Read the model definition and answer for the solid it produces. Units are mm, in the model's axes. A direction names the side the tool comes from. Coordinates: 2 decimals unless noted, no trailing zeros. Loops run counter-clockwise (first coordinate to the right, second up) from the corner with the lowest first, then second, coordinate; pieces in that order, holes last. Notation, with made-up numbers: M 13,27 L 45,27 A21 ccw 45,32 Z; hole C 34,39 d3. An arc over 180 degrees is marked long. Put each result on its own line as item: value.
from build123d import *

# Parameters (mm, degrees)
CROQUIS1_R              = 11
CROQUIS1_R_2            = 6
SALIENTE_EXTRUIR1_DEPTH = 25
CROQUIS2_W              = 6
CROQUIS2_H              = 22
CORTAR_EXTRUIR1_DEPTH   = 25
CROQUIS3_R              = 11
CROQUIS3_R_2            = 8.5
SALIENTE_EXTRUIR2_DEPTH = 25
SALIENTE_EXTRUIR3_DEPTH = 10
SALIENTE_EXTRUIR4_DEPTH = 10
CROQUIS9_R              = 11
CROQUIS9_R_2            = 8.5
SALIENTE_EXTRUIR5_DEPTH = 10
CROQUIS13_R             = 11
CROQUIS13_R_2           = 6
SALIENTE_EXTRUIR6_DEPTH = 5
CROQUIS14_W             = 6
CROQUIS14_H             = 22
CORTAR_EXTRUIR2_DEPTH   = 5
CROQUIS15_R             = 11
CROQUIS15_R_2           = 8.5
SALIENTE_EXTRUIR7_DEPTH = 5


with BuildPart() as part:
    # Croquis1 → Saliente-Extruir1 (new body)
    with BuildSketch(Plane.XY):
        Circle(CROQUIS1_R)
        Circle(CROQUIS1_R_2, mode=Mode.SUBTRACT)
    extrude(amount=SALIENTE_EXTRUIR1_DEPTH)

    # Croquis2 → Cortar-Extruir1 (cut)
    with BuildSketch(Plane.XY.offset(25)):
        Rectangle(CROQUIS2_W, CROQUIS2_H)
    extrude(amount=-CORTAR_EXTRUIR1_DEPTH, mode=Mode.SUBTRACT)

    # Croquis3 → Saliente-Extruir2 (add)
    with BuildSketch(Plane.XY):
        Circle(CROQUIS3_R)
        Circle(CROQUIS3_R_2, mode=Mode.SUBTRACT)
    extrude(amount=SALIENTE_EXTRUIR2_DEPTH)

    # Croquis4 → Saliente-Extruir3 (add)
    with BuildSketch(Plane.XY.offset(25)):
        with BuildLine():
            Line((3, 5.196152423), (3, 10.583005244))
            ThreePointArc((3, 10.583005244), (5.366490611, 9.602123647), (7.441930866, 8.100473133))
            Line((7.441930866, 8.100473133), (4.059235018, 4.418439891))
            ThreePointArc((4.059235018, 4.418439891), (3.550972959, 4.83638202), (3, 5.196152423))
        make_face()
    extrude(amount=SALIENTE_EXTRUIR3_DEPTH)

    # Croquis8 → Saliente-Extruir4 (add)
    with BuildSketch(Plane.XY.offset(25)):
        Polygon((-3, -10.583005244), (-3, -5.196152423), (-3.883308042, -4.573829758), (-7.119398076, -8.385354556), align=None)
    extrude(amount=SALIENTE_EXTRUIR4_DEPTH)

    # Croquis9 → Saliente-Extruir5 (add)
    with BuildSketch(Plane.XY.offset(25)):
        Circle(CROQUIS9_R)
        Circle(CROQUIS9_R_2, mode=Mode.SUBTRACT)
    extrude(amount=SALIENTE_EXTRUIR5_DEPTH)

    # Croquis13 → Saliente-Extruir6 (add)
    with BuildSketch(Plane(origin=(0, 0, 0), x_dir=(-1, 0, 0), z_dir=(0, 0, -1))):
        Circle(CROQUIS13_R)
        Circle(CROQUIS13_R_2, mode=Mode.SUBTRACT)
    extrude(amount=SALIENTE_EXTRUIR6_DEPTH)

    # Croquis14 → Cortar-Extruir2 (cut)
    with BuildSketch(Plane(origin=(0, 0, -5), x_dir=(-1, 0, 0), z_dir=(0, 0, -1))):
        Rectangle(CROQUIS14_W, CROQUIS14_H)
    extrude(amount=-CORTAR_EXTRUIR2_DEPTH, mode=Mode.SUBTRACT)

    # Croquis15 → Saliente-Extruir7 (add)
    with BuildSketch(Plane(origin=(0, 0, -5), x_dir=(-1, 0, 0), z_dir=(0, 0, -1))):
        Circle(CROQUIS15_R)
        Circle(CROQUIS15_R_2, mode=Mode.SUBTRACT)
    extrude(amount=-SALIENTE_EXTRUIR7_DEPTH)


solid = part.part
1) Find section B-B, the plane x = 0. Write down the section's boundary in (y, z).
Answer list:
outline: M -11,-5 L -8.5,-5 L -8.5,35 L -11,35 Z; M 8.5,-5 L 11,-5 L 11,35 L 8.5,35 Z
2) Find section C-C, the plane y = -2.5. Write down the section's boundary in (x, z), plus the area to 3 significant figures.
Answer list:
outline: M -10.71,-5 L -5.45,-5 L -5.45,25 L -8.12,25 L -8.12,35 L -10.71,35 Z; M 5.45,-5 L 10.71,-5 L 10.71,35 L 8.12,35 L 8.12,25 L 5.45,25 Z
area: 367 mm^2
3) Find section D-D, the plane z = 7. Write down the section's boundary in (x, y).
Answer list:
outline: C 0,0 d22; hole M -3,-7.95 A8.5 ccw 3,-7.95 L 3,-5.2 A6 ccw 3,5.2 L 3,7.95 A8.5 ccw -3,7.95 L -3,5.2 A6 ccw -3,-5.2 Z
4) Which of the six approach directions +Z, -Z, +X, -X, +Y, -Y give full straight-line access (tool end or side, diameter ignored) to faces 1 (the flat face through (4.917, 5.352, 29.93)), 2 (the flat face through (-3.435, -4.889, 29.93))?
Answer list:
face 1: +Z
face 2: +Z, -Z
5) Given pin 1 Ø4 at (x, y) = (0.5, 4.5) entering from -Z; pin 2 Ø3 at (y, z) = (7, 6.5) entering from +X; pin 3 Ø1.7 at (x, y) = (-5, 2.5) entering from +Z; pin 4 Ø1.4 at (y, z) = (-6.5, 17.5) entering from -X, each flat-ended and moving along its own axis, determine where each tip first touches the part or whether it passes through.
Answer list:
pin 1: passes through
pin 2: stops at x = 9.53
pin 3: stops at z = 25
pin 4: stops at x = -9.35
6) Determine the mould class of faces 3 (the flat face through (6.3, -0.7, 25)), 4 (the flat face through (4, 6, 35)) for opening direction Y: released by +Y, released by -Y, zero draft, split by the parting line, or undercut.
Answer list:
face 3: undercut
face 4: zero draft
7) Find section A-A, the plane z = 25.5. Write down the section's boundary in (x, y).
Answer list:
outline: C 0,0 d22; hole M -5.5,-6.48 L -3.88,-4.57 L -3,-5.2 L -3,-7.95 A8.5 ccw 5.75,6.26 L 4.06,4.42 A6 ccw 3,5.2 L 3,7.95 A8.5 ccw Z
8) Straight lines are drawn through the part: line 1 (Y direction, x = 0.25, z = 4); line 2 (Z direction, x = 3.25, y = -7); line 3 (Y direction, x = -2, z = 13.5). For each, find the intervals that lie inside material, in ascending order. Write a range as [from, to].
Answer list:
line 1: y = [-11, -8.5], [8.5, 11]
line 2: z = [-5, 25]
line 3: y = [-10.82, -8.26], [8.26, 10.82]
